Autodesk Inventor part; units mm, degrees
ref_plane "YZ Plane" through (0, 0, 0) normal (1, 0, 0) x (0, 1, 0)
ref_plane "XZ Plane" through (0, 0, 0) normal (0, 1, 0) x (-1, 0, 0)
ref_plane "XY Plane" through (0, 0, 0) normal (0, 0, 1) x (1, 0, 0)
sketch "Sketch1" plane through (0, 0, 0) normal (0, 0, 1) x (1, 0, 0)
  line L0 (0, 0) -> (101.6, 0)
  line L1 (101.6, 0) -> (101.6, 76.2)
  line L2 (101.6, 76.2) -> (0, 76.2)
  line L3 (0, 76.2) -> (0, 0)
  dimension "d0" = 101.6
  dimension "d1" = 76.2
extrude "Extrusion1" add sketch "Sketch1" along normal blind 76.2
sketch "Sketch2" plane through (0, 76.2, 0) normal (0, 1, 0) x (1, 0, 0)
  line L0 (101.6, 0) -> (101.6, -76.2)
  line L1 (101.6, -19.812) -> (66.04, -19.812)
  line L2 (66.04, -19.812) -> (66.04, -56.388)
  line L3 (66.04, -56.388) -> (101.6, -56.388)
  line L4 (101.6, -56.388) -> (101.6, -19.812)
  point P0 (0, 0)
  dimension "d4" = 35.56
  dimension "d5" = 36.576
  dimension "d6" = 19.812
extrude "Extrusion2" cut sketch "Sketch2" against normal blind 76.2
sketch "Sketch3" plane through (0, 0, 76.2) normal (0, 0, 1) x (1, 0, 0)
  line L0 (0, 75.8832) -> (15.9989, 76.2)
  line L1 (101.6, 76.2) -> (0, 76.2)
  line L2 (66.04, 0) -> (101.6, 0)
  line L3 (101.6, 0) -> (50.8, 0)
  line L4 (101.6, 0) -> (101.6, 38.1)
  line L5 (101.6, 76.2) -> (101.6, 0)
  line L6 (50.8, 0) -> (50.8, 38.1)
  line L7 (15.9989, 76.2) -> (50.8, 38.1)
  line L8 (101.6, 38.1) -> (101.6, 90.7152)
  line L9 (101.6, 90.7152) -> (15.9989, 90.7152)
  line L10 (15.9989, 90.7152) -> (15.9989, 76.2)
  line L11 (50.8, 38.1) -> (101.6, 38.1)
  point P0 (0, 0)
  dimension "d9" = 16.002
  dimension "d10" = 50.8
  dimension "d11" = 38.1
extrude "Extrusion3" cut sketch "Sketch3" against normal blind 76.2 contours L5 L11 L7 L1
sketch "Sketch4" plane through (101.6, 0, 76.2) normal (1, 0, 0) x (0, 0, -1)
  line L0 (76.2, 38.1) -> (56.388, 38.1)
  line L1 (0, 0) -> (0, 38.1)
  line L2 (76.2, 38.1) -> (0, 38.1)
  line L3 (0, 38.1) -> (0, 14.224)
  line L4 (0, 14.224) -> (76.2, 38.1)
  point P0 (76.2, 0)
  dimension "d14" = 23.876
extrude "Extrusion4" cut sketch "Sketch4" against normal blind 50.8
sketch "Sketch5" plane through (0, 0, 0) normal (-1, 0, 0) x (0, 0, 1)
  point P0 (0, 0)
sketch "Sketch6" plane through (0, 0, 0) normal (-1, 0, 0) x (0, 0, 1)
  point P0 (0, 0)
sketch "Sketch7" plane through (0, 0, 0) normal (-1, 0, 0) x (0, 0, 1)
  line L0 (76.2, 76.2) -> (0, 76.2)
  line L1 (63.5, 76.2) -> (38.1, 76.2)
  line L2 (38.1, 76.2) -> (38.1, 52.324)
  line L3 (38.1, 52.324) -> (63.5, 76.2)
  line L4 (12.7, 76.2) -> (38.1, 76.2)
  line L5 (38.1, 52.324) -> (12.7, 76.2)
  line L6 (12.7, 76.2) -> (63.5, 76.2)
  point P0 (0, 0)
  dimension "d17" = 25.4
  dimension "d18" = 23.876
  dimension "d19" = 12.7
sketch "Sketch8" plane through (0, 0, 0) normal (-1, 0, 0) x (0, 0, 1)
  point P0 (0, 0)
extrude "Extrusion5" cut sketch "Sketch7" against normal blind 50.8
properties part number "orthographic2"
Model file for the job. Use its own axes, mm. A direction names the side the tool comes from. Coordinates: 2 decimals unless noted, no trailing zeros. Loops run counter-clockwise (first coordinate to the right, second up) from the corner with the lowest first, then second, coordinate; pieces in that order, holes last. Notation, with made-up numbers: (-8.75, 34.5) -> (36.25, 34.5) arc R32 cw to (36.25, 64.5) -> close; hole circle Ø2 at (49.5, -33.5). An arc over 180 degrees is marked (long way). Answer as a JSON object with one key per item and string values.
Q1. Cut at A-A (x = 89). List the corners of the cut face in (y, z), and give its area (3 significant figures).
Report:
{"outline": "(0, 0) -> (38.1, 0) -> (31.89, 19.81) -> (0, 19.81) -> close; (0, 56.39) -> (20.43, 56.39) -> (14.22, 76.2) -> (0, 76.2) -> close", "area": "1,040 mm2"}
Q2. Flat gauge pins, fed straight in: P1, Ø8, axis at x = 61, z = 43.5, coming from the +Y side; P2, Ø1, axis at x = 67, z = 63, coming from the +Y side; P3, Ø2, axis at y = 45, z = 21, coming from the +X side. Where does each tip first touch, or does it go through?
Report:
{"P1": "stops at y = 25.72", "P2": "stops at y = 18.52", "P3": "stops at x = 45.41"}
Q3. Cut at B-B (y = 61.5). List the corners of the cut face in (x, z).
Report:
{"outline": "(0, 0) -> (29.43, 0) -> (29.43, 28.34) -> (0, 28.34) -> close; (0, 47.86) -> (29.43, 47.86) -> (29.43, 76.2) -> (0, 76.2) -> close"}
Q4. Probe probe 1 along X at (y, z) = (25.5, 48.5); probe 2 along X at (y, z) = (19, 42); probe 3 along Z at (x, y) = (82, 28). List the from-to ranges inside material, lowest first.
Report:
{"probe 1": "x = 0 to 50.8", "probe 2": "x = 0 to 66.04", "probe 3": "z = 0 to 19.81"}
Q5. Cut at D-D (z = 68). List the corners of the cut face in (x, y), and give its area (3 significant figures).
Report:
{"outline": "(0, 0) -> (101.6, 0) -> (101.6, 16.79) -> (50.8, 16.79) -> (50.8, 38.1) -> (16, 76.2) -> (0, 76.2) -> close", "area": "4,060 mm2"}
Q6. 3-axis set-ups, long thin cutter, end or side, ignore diameter. For faces 5 (the flat face through (8, 76.2, 70)), 6 (the flat face through (84, 10, 56.388)), 7 (the flat face through (50.8, 29, 47)), 8 (the flat face through (14.44, 61.44, 47.8)), 9 (the flat face through (39, 30, 76.2)): which of +Z, -Z, +X, -X, +Y, -Y reach the whole face in a straight line?
Report:
{"face 5": "+Z, -Z, +X, -X, +Y", "face 6": "+X, +Y, -Y", "face 7": "+Z, +X, +Y", "face 8": "+X, -X, +Y", "face 9": "+Z, +X, -X, +Y, -Y"}
Q7. Pull direction Z, two halves, no side cores. Call faces 1 (the flat face through (39, 30, 0)), 2 (the flat face through (65.267, 25.995, 38.633)), 3 (the flat face through (39, 0, 38)), 4 (the flat face through (84, 16, 19.812)): released by +Z, released by -Z, zero draft, split by the parting line, or undercut.
Report:
{"face 1": "released by -Z", "face 2": "released by +Z", "face 3": "zero draft", "face 4": "undercut"}
Q8. Cut at C-C (x = 10). List the corners of the cut face in (y, z).
Report:
{"outline": "(0, 0) -> (76.2, 0) -> (76.2, 12.7) -> (52.32, 38.1) -> (76.2, 63.5) -> (76.2, 76.2) -> (0, 76.2) -> close"}
